Source: CAD feature listing. Evaluate the final solid. Frame: model axes, mm. A direction names the side the tool comes from. Coordinates: 2 decimals unless noted, no trailing zeros. One line per question, with ' | ' between items.
from build123d import *

# Parameters (mm, degrees)
BOSS_EXTRUDE1_DEPTH = 2.54
EXTRUDE_THIN1_DEPTH = 38.1


# Read off the part's stored shape, not the designer's step: Extrude-Thin1
with BuildPart() as part:
    # Sketch60 → Boss-Extrude1 (new body)
    with BuildSketch(Plane(origin=(0, 0, 0), x_dir=(0, 0, -1), z_dir=(1, 0, 0))):
        with BuildLine():
            Line((1327.15, 331.787470833), (1327.15, 382.587350833))
            Line((1327.15, 382.587350833), (1377.950002406, 382.587350833))
            Line((1377.950002406, 382.587350833), (1377.950002406, 350.761150833))
            Line((1377.950002406, 350.761150833), (1363.014798129, 350.761150833))
            ThreePointArc((1363.014798129, 350.761150833), (1354.048599065, 359.727349897), (1345.0824, 350.761150833))
            Line((1345.0824, 350.761150833), (1345.0824, 338.838562796))
            ThreePointArc((1345.0824, 338.838562796), (0, -382.587529167), (-1345.0824, 338.838562795))
            Line((-1345.0824, 338.838562795), (-1345.0824, 350.761150833))
            ThreePointArc((-1345.0824, 350.761150833), (-1354.048599065, 359.727349897), (-1363.014798129, 350.761150833))
            Line((-1363.014798129, 350.761150833), (-1377.950002406, 350.761150833))
            Line((-1377.950002406, 350.761150833), (-1377.950002406, 382.587350833))
            Line((-1377.950002406, 382.587350833), (-1327.15, 382.587350833))
            Line((-1327.15, 382.587350833), (-1327.15, 331.787470833))
            add(Edge.make_bspline(
                [(1327.15, 331.787470833), (1e-09, -995.362529167), (-1327.15, 331.787470833)],
                knots=[0, 0, 0, 1, 1, 1], degree=2))
        make_face()
    extrude(amount=BOSS_EXTRUDE1_DEPTH)

    # Extrude-Thin1 outline → Extrude-Thin1 (add)
    with BuildSketch(Plane(origin=(2.54, 0, 0), x_dir=(0, 0, -1), z_dir=(1, 0, 0))):
        with BuildLine():
            add(Edge.make_bspline(
                [(1331.64012806, 327.297342772), (1220.857206072, 216.514420784), (1110.039266695, 119.543483359), (888.305733392, -46.756666627), (777.389280582, -116.086154697), (555.440332256, -227.060628875), (444.406603679, -268.704745917), (222.248599022, -324.244247103), (111.125000161, -338.137529152), (-111.124999809, -338.137529182), (-222.24859867, -324.244247162), (-444.406603328, -268.704746034), (-555.440331905, -227.060629021), (-777.389280231, -116.086154902), (-888.305733041, -46.756666861), (-1110.039266345, 119.543483066), (-1220.857205722, 216.514420463), (-1331.64012771, 327.297342421)],
                knots=[0, 0, 0, 0, 0.125, 0.125, 0.25, 0.25, 0.375, 0.375, 0.5, 0.5, 0.625, 0.625, 0.75, 0.75, 0.875, 0.875, 1, 1, 1, 1], degree=3))
            Line((1331.64012806, 327.297342772), (1333.5, 331.787470833))
            Line((1333.5, 331.787470833), (1333.5, 382.587350833))
            Line((1333.5, 382.587350833), (1332.23, 382.587350833))
            Line((1332.23, 382.587350833), (1332.23, 332.04008954))
            Line((1332.23, 332.04008954), (1330.563482535, 328.016760475))
            add(Edge.make_bspline(
                [(1330.563482535, 328.016760475), (1219.832830837, 217.300990844), (1109.074174075, 120.39600204), (887.478733858, -45.778240912), (776.641272659, -115.047704785), (554.873550579, -225.916661245), (443.942272952, -267.515471252), (222.0073883, -322.991733554), (111.004224806, -336.867529153), (-111.004224472, -336.867529181), (-222.007387967, -322.991733609), (-443.942272618, -267.515471364), (-554.873550246, -225.916661384), (-776.641272326, -115.047704979), (-887.478733526, -45.778241134), (-1109.074173743, 120.396001763), (-1219.832830505, 217.300990539), (-1330.563482203, 328.016760142)],
                knots=[0, 0, 0, 0, 0.125, 0.125, 0.25, 0.25, 0.375, 0.375, 0.5, 0.5, 0.625, 0.625, 0.75, 0.75, 0.875, 0.875, 1, 1, 1, 1], degree=3))
            Line((-1330.563482203, 328.016760142), (-1332.23, 332.040089565))
            Line((-1332.23, 332.040089565), (-1332.23, 382.587350833))
            Line((-1332.23, 382.587350833), (-1333.5, 382.587350833))
            Line((-1333.5, 382.587350833), (-1333.5, 331.787470833))
            Line((-1333.5, 331.787470833), (-1331.64012771, 327.297342421))
        make_face()
    extrude(amount=EXTRUDE_THIN1_DEPTH)


solid = part.part
(1) Set-up query: faces 1 (the flat face through (2.54, -338.3, -6.4)), 2 (the cylindrical face through (1.252, -382.434, -22.256)). Return all of +Z, -Z, +X, -X, +Y, -Y with unobstructed straight access to the full face (end or side cutting, diameter ignored); none if empty.
Taken from the geometry:
face 1: +X, -Y | face 2: +X, -X, -Y
(2) Pin query (flat end, axial travel): P1, Ø8, axis at x = 34.5, y = -136, coming from the -Z side; P2, Ø10, axis at x = 14, y = 72, coming from the +Z side; P3, Ø3, axis at x = 21.5, z = -867.5, coming from the -Y side. Return the tip coordinate at first contact, or that it passes through.
Taken from the geometry:
P1: stops at z = -741.35 | P2: stops at z = 1051.92 | P3: stops at y = -56.82
(3) Material intervals for L1, parallel to Z at x = 11, y = 334; L2, parallel to Z at x = 20, y = 180; L3, parallel to Y at x = 10.5, z = -497, sorted ascending. Write a range as from..to.
Taken from the geometry:
L1: z = -1333.5..-1332.23, 1332.23..1333.5 | L2: z = -1175.13..-1173.21, 1173.21..1175.13 | L3: y = -245.51..-244.15
